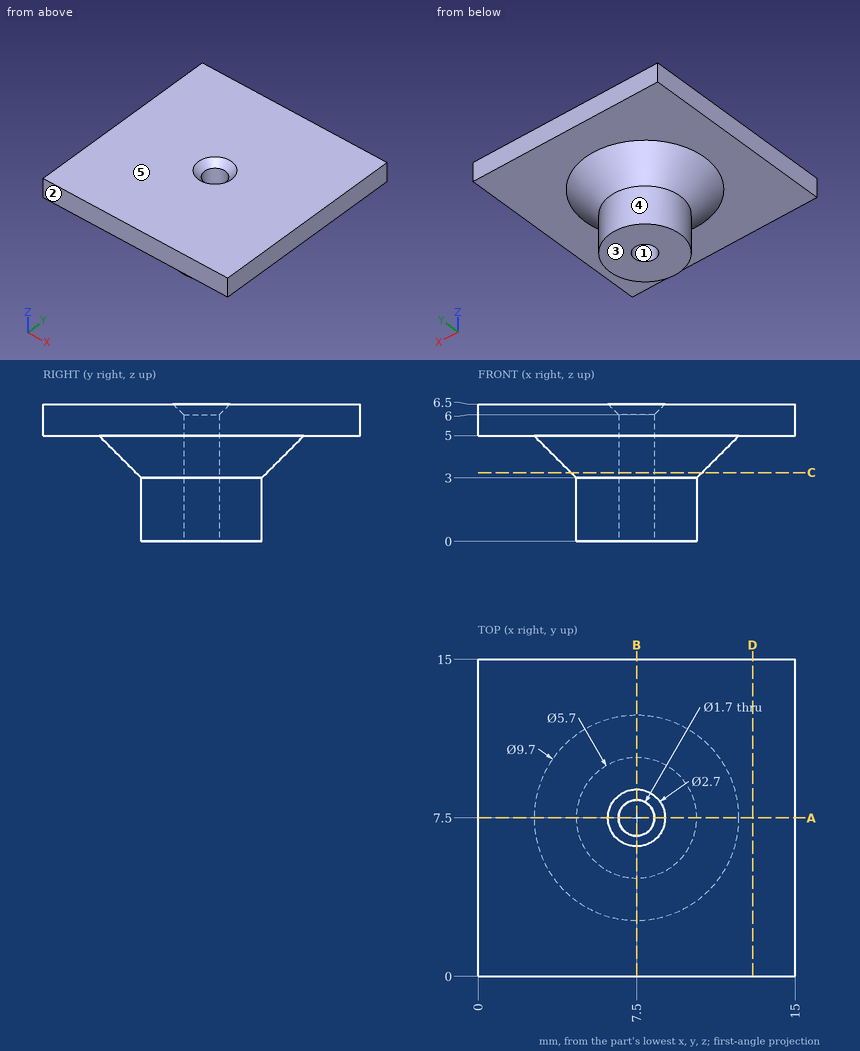
The drawing under review shows one solid part. Ordinate dimensions are in mm from its lowest x, y, z. A direction names the side the tool comes from. Coordinates: 2 decimals unless noted, no trailing zeros. Order: outer loops, then holes, each group sorted by start corner. A loop starts at its lowest first (then second) coordinate and runs counter-clockwise, first axis right, second up. Notation, with made-up numbers: (82, 64) -> (110, 64) arc R25 ccw to (110, 78) -> close; hole circle Ø9 at (-6, 73). An arc over 180 degrees is marked (long way). One line per item, written item: value.
1) We need section D-D, the plane x = 13. Give the boundary of the cut face in (y, z).
Output values:
outline: (0, 5) -> (15, 5) -> (15, 6.5) -> (0, 6.5) -> close
2) To check wall thickness, follow probe 1 along Y at (x, z) = (7.5, 1.3); probe 2 along Z at (x, y) = (5.25, 1.75); probe 3 along Y at (x, z) = (7.5, 3.5). State the ranges of each line that lie inside material, in increasing order. Write a range as [from, to].
Output values:
probe 1: y = [4.65, 6.65], [8.35, 10.35]
probe 2: z = [5, 6.5]
probe 3: y = [4.15, 6.65], [8.35, 10.85]
3) We need section A-A, the plane y = 7.5. Give the boundary of the cut face in (x, z).
Output values:
outline: (0, 5) -> (2.65, 5) -> (4.65, 3) -> (4.65, 0) -> (6.65, 0) -> (6.65, 6) -> (6.15, 6.5) -> (0, 6.5) -> close; (8.35, 0) -> (10.35, 0) -> (10.35, 3) -> (12.35, 5) -> (15, 5) -> (15, 6.5) -> (8.85, 6.5) -> (8.35, 6) -> close
4) Draft analysis for pull direction Y (two halves, no side actions). For the marked faces 1, 2 and 3, state which applies: +Y half, -Y half, draft (parallel to the pull), parting line (faces both ways), or undercut.
Output values:
face 1: undercut
face 2: -Y half
face 3: draft
5) We need section C-C, the plane z = 3.25. Give the boundary of the cut face in (x, y), then the cut area to 3 significant figures.
Output values:
outline: circle Ø6.2 at (7.5, 7.5); hole circle Ø1.7 at (7.5, 7.5)
area: 27.9 mm2
6) Clearance check with flat-ended pins moving along their axes: P1, Ø2, axis at y = 5.5, z = 2, coming from the +X side; P2, Ø3, axis at x = 11, y = 12, coming from the -Z side; P3, Ø5, axis at x = 10.5, y = 2.5, coming from the -Z side. State where each tip first meets the part, or that it passes through.
Output values:
P1: stops at x = 10.17
P2: stops at z = 4.35
P3: stops at z = 3.48
7) Machinability: for the marked faces 4 and 5, which of the approach directions +Z, -Z, +X, -X, +Y, -Y give a long, thin tool a straight path to every point of the face, cutting with its end or side? Answer none if there is none.
Output values:
face 4: -Z
face 5: +Z, +X, -X, +Y, -Y
